Check sheet for the drawn part. Datum: minimum x, y, z corner. Units: mm. A direction names the side the tool comes from. Round coordinates to 2 decimals unless told otherwise and drop trailing zeros. Order: outer loops, then holes, each group sorted by start corner. A loop starts at its lowest first (then second) coordinate and runs counter-clockwise, first axis right, second up. Notation, with made-up numbers: M 58,46 L 108,46 A5 ccw 108,52 Z; hole C -36,38.25 d9. An arc over 180 degrees is marked long. Use one line per item in the form item = value. Start each with the question number.
Item 1: Thickness scan on probe 1 along Z at (x, y) = (28, 3.75); probe 2 along X at (y, z) = (3.25, 14); probe 3 along Z at (x, y) = (28, 2.75). Record the ranges inside material, lowest first. Write a range as [from, to].
Item 2: Cross-section at D-D on z = 36.5. Enter the section's corners in (x, y).
Item 3: Go/stop test with a flat-tipped pin: pin 1 Ø1 at (x, z) = (48, 37.5) entering from +Y. Record where the tip stops, or that it passes through.
Item 4: Release check for a two-part mould opening along X. For the marked faces 3, 4 and 5 record: +X half, -X half, draft (parallel to the pull), parting line (faces both ways), or undercut.
Item 5: Tool access check on the marked faces 1 and 2. Record the directions out of +Z, -Z, +X, -X, +Y, -Y that give a thin tool (end or side, any length) a straight path to the whole face; none if there is none.
Item 6: Cross-section at A-A on y = 5.5. Enter the section's corners in (x, z), then the cut area to 3 significant figures.
Item 7: Cross-section at C-C on x = 28. Enter the section's corners in (y, z).
Item 8: Cross-section at B-B on z = 14.5. Enter the section's corners in (x, y), then the cut area to 4 significant figures.
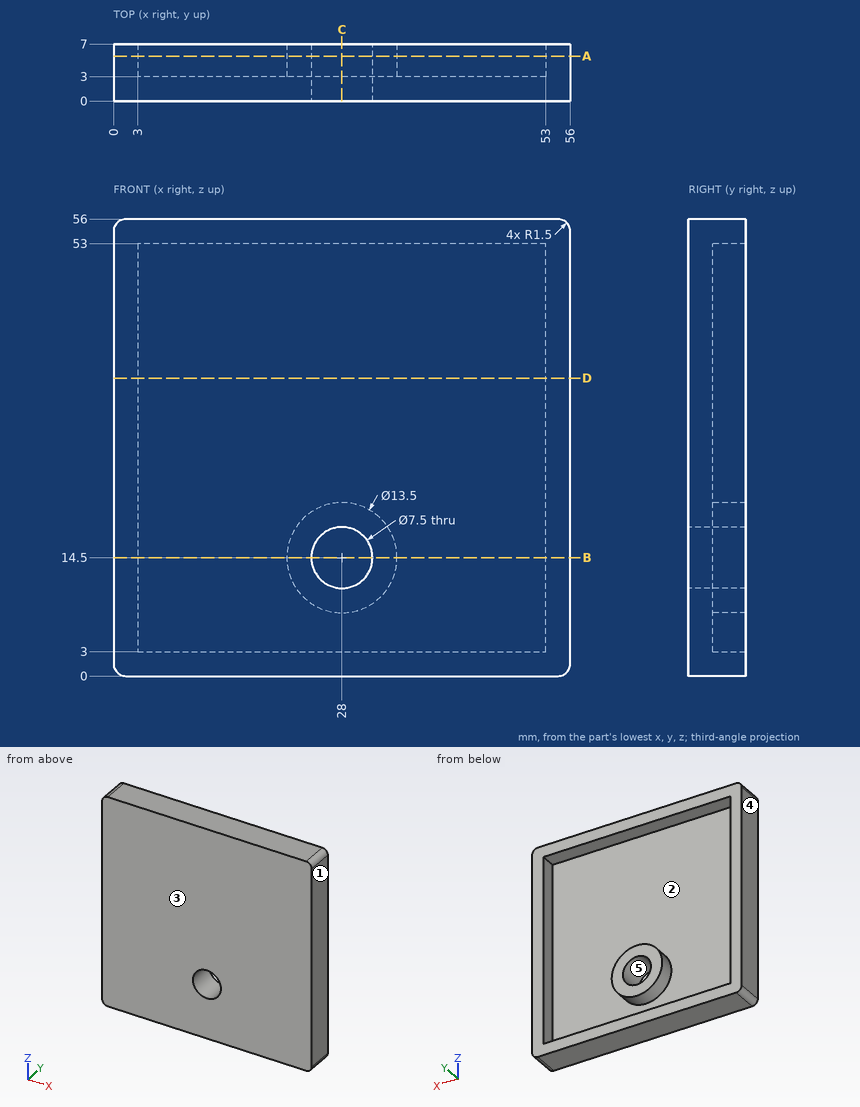
Output values:
q1.probe_1 = [0, 3], [7.75, 10.75], [18.25, 21.25], [53, 56]
q1.probe_2 = [0, 3], [21.27, 24.28], [31.72, 34.73], [53, 56]
q1.probe_3 = [0, 10.75], [18.25, 56]
q2.outline = M 0,0 L 56,0 L 56,7 L 53,7 L 53,3 L 3,3 L 3,7 L 0,7 Z
q3.pin_1 = 3
q4.face_3 = draft
q4.face_4 = -X half
q4.face_5 = undercut
q5.face_1 = +Z, -Z, +X, +Y, -Y
q5.face_2 = +Y
q6.outline = M 0,1.5 A1.5 ccw 1.5,0 L 54.5,0 A1.5 ccw 56,1.5 L 56,54.5 A1.5 ccw 54.5,56 L 1.5,56 A1.5 ccw 0,54.5 Z; C 28,14.5 d13.5; hole M 3,3 L 53,3 L 53,53 L 3,53 Z; hole C 28,14.5 d7.5
q6.area = 733 mm2
q7.outline = M 0,0 L 7,0 L 7,3 L 3,3 L 3,7.75 L 7,7.75 L 7,10.75 L 0,10.75 Z; M 0,18.25 L 7,18.25 L 7,21.25 L 3,21.25 L 3,53 L 7,53 L 7,56 L 0,56 Z
q8.outline = M 0,0 L 24.25,0 L 24.25,7 L 21.25,7 L 21.25,3 L 3,3 L 3,7 L 0,7 Z; M 31.75,0 L 56,0 L 56,7 L 53,7 L 53,3 L 34.75,3 L 34.75,7 L 31.75,7 Z
q8.area = 193.5 mm2
